Read the model definition and answer for the solid it produces. Units are mm, in the model's axes. Round coordinates to 2 decimals unless told otherwise and drop trailing zeros. Write each loop counter-clockwise with the first axis right and the second up, starting at its lowest first coordinate (ties: lowest second). Pieces come first, ordered by that corner, then holes. Notation, with made-up numbers: (-35.5, -8.5) -> (-10.5, -8.5) arc R11 cw to (-10.5, 1.5) -> close; hole circle Ø9 at (-40, -29.75). An arc over 180 degrees is marked (long way). Return JSON: item names as keys, results as strings. Group by question number.
(1) A cutting plane is placed at B-B on y = 1.7. State how many separate pieces and enclosed holes the cut face has, then the cut area to 3 significant figures.
(2) A cutting plane is placed at A-A on z = -48.5. Give the vertices of the cut face in (x, y).
(3) A cutting plane is placed at C-C on x = 75. Give the vertices of the cut face in (y, z).
(4) Straight lines are drawn through the part: line 1 (X direction, y = 2.4, z = -90); line 2 (X direction, y = 0.9, z = -183); line 3 (Z direction, x = 91, y = 2.5). For each, find the intervals that lie inside material, in ascending order.
(5) A cutting plane is placed at D-D on x = 255.5. Give the vertices of the cut face in (y, z), then the cut area to 3 significant figures.
(6) The mould has two halves that part along Z. Classify faces 1 (the flat face through (55.536, 1.377, -97.562)), 2 (the flat face through (153, 2.794, -76)), 3 (the cylindrical face through (128.087, 1.377, -96.48)): released by +Z, released by -Z, zero draft, split by the parting line, or undercut.
Autodesk Fusion 360 part; units mm, degrees
sketch "Sketch1" plane through (0, 0, 0) normal (0, 1, 0) x (1, 0, 0)
  line L0 (0, 0) -> (310.515, 0)
  line L1 (155.2575, 192.4304) -> (109.5375, 192.4304)
  line L2 (155.2575, 192.4304) -> (200.9775, 192.4304)
  line L3 (200.9775, 192.4304) -> (310.515, 0)
  line L4 (109.5375, 192.4304) -> (0, 0)
  circle A0 centre (155.2575, 96.8375) radius 8.128
  circle A1 centre (174.3075, 70.1675) radius 1.9812
  circle A2 centre (174.3075, 112.3315) radius 1.9812
  circle A3 centre (155.2575, 41.275) radius 11.1125
  circle A4 centre (136.2075, 96.8375) radius 8.128
  circle A5 centre (155.2575, 70.1675) radius 1.9812
  circle A6 centre (136.2075, 70.1675) radius 1.9812
  circle A7 centre (174.3075, 96.8375) radius 8.128
  circle A8 centre (136.2075, 112.3315) radius 1.9812
  circle A9 centre (155.2575, 112.3315) radius 1.9812
  circle A10 centre (27.0579, 21.862) radius 1.905
  circle A11 centre (86.334, 125.9954) radius 1.905
  circle A12 centre (45.2777, 53.8696) radius 1.905
  circle A13 centre (129.8575, 164.4904) radius 1.905
  circle A14 centre (129.8575, 182.2704) radius 1.905
  circle A15 centre (104.5538, 158.0031) radius 1.905
  circle A16 centre (224.181, 125.9954) radius 1.905
  circle A17 centre (265.2373, 53.8696) radius 1.905
  circle A18 centre (180.6575, 182.2704) radius 1.905
  circle A19 centre (283.4571, 21.862) radius 1.905
  circle A20 centre (180.6575, 164.4904) radius 1.905
  circle A21 centre (205.9612, 158.0031) radius 1.905
  point P0 (104.5538, 158.0031)
  point P1 (205.9612, 158.0031)
  dimension "d1" = 310.515
  dimension "d3" = 45.72
  dimension "d4" = 45.72
  dimension "d45" = 22.225
  dimension "d46" = 16.256
  dimension "d47" = 26.67
  dimension "d48" = 3.9624
  dimension "d49" = 42.164
  dimension "d50" = 3.9624
  dimension "d51" = 16.256
  dimension "d52" = 26.67
  dimension "d53" = 3.9624
  dimension "d54" = 42.164
  dimension "d55" = 3.9624
  dimension "d56" = 16.256
  dimension "d57" = 26.67
  dimension "d58" = 3.9624
  dimension "d59" = 42.164
  dimension "d60" = 3.9624
extrude "Extrude5" add sketch "Sketch1" along normal blind 2.794
extrude "Extrude4" [suppressed]
equation "d3 = ( 3.6 / 2 ) * 1 in"
equation "d4 = ( 3.6 / 2 ) * 1 in"
Checks:
{
 "1": {"separate pieces": "1", "enclosed holes": "22", "area": "37,500 mm^2"},
 "2": {"outline": "(27.61, 0) -> (146.81, 0) -> (146.81, 2.79) -> (27.61, 2.79) -> close; (163.7, 0) -> (282.91, 0) -> (282.91, 2.79) -> (163.7, 2.79) -> close"},
 "3": {"outline": "(0, -131.76) -> (2.79, -131.76) -> (2.79, 0) -> (0, 0) -> close"},
 "4": {"line 1": "x = 51.23 to 131.81, 140.6 to 150.86, 159.65 to 169.91, 178.7 to 259.28", "line 2": "x = 104.17 to 128.1, 131.62 to 178.9, 182.42 to 206.35", "line 3": "z = -159.86 to 0"},
 "5": {"outline": "(0, -96.65) -> (2.79, -96.65) -> (2.79, 0) -> (0, 0) -> close", "area": "270 mm^2"},
 "6": {"face 1": "released by -Z", "face 2": "zero draft", "face 3": "undercut"}
}
